Input: part model. Units: mm. Frame: model coordinates. Coordinates: 2 decimals unless noted, no trailing zeros. Order: outer loops, then holes, each group sorted by start corner. A loop starts at its lowest first (then second) coordinate and runs counter-clockwise, first axis right, second up.
from build123d import *

# Parameters (mm, degrees)
F0_W     = 25.4
F0_H     = 25.4
F2_R     = 19.05
F3_SIZE2 = 2.961044
F3_SIZE  = 6.34999


# Not quite as in the source:
# - a fillet or chamfer is up to 0.001 mm smaller than in the source, because OpenCascade refuses the exact size


with BuildPart() as f1:
    # F0 (on Front) → F1 (revolve)
    with BuildSketch(Plane.XZ):
        with Locations((12.7, 12.7)):
            Rectangle(F0_W, F0_H)
    revolve(axis=Axis((0, 0, 12.7), (0, 0, 1)))

    # F2
    f2_edges = [f1.edges().sort_by_distance(p)[0] for p in [
        (-25.4, 0, 25.4),
    ]]
    fillet(f2_edges, radius=F2_R)

    # F3 (size 6.35 and 2.9610536293 in the source; OpenCascade refuses exactly that, so slightly less here)
    f3_edges = [f1.edges().sort_by_distance(p)[0] for p in [
        (-25.4, 0, 0),
    ]]
    chamfer(f3_edges, length=F3_SIZE, length2=F3_SIZE2)


solid = f1.part
Item 1: Pin query (flat end, axial travel): pin 1 Ø2 at (x, z) = (-18.5, 17.5) entering from +Y; pin 2 Ø6 at (x, y) = (9, 8) entering from +Z; pin 3 Ø1 at (y, z) = (3.5, 6) entering from -X. Return the tip coordinate at first contact, or that it passes through.
Response values:
pin 1: stops at y = 13.42
pin 2: stops at z = 25.21
pin 3: stops at x = -25.2
Item 2: Cut plane A-A on z = 3.5. Return loops of the section in (x, y).
Response values:
outline: circle Ø48.14 at (0, 0)
Item 3: Ray query, probe 1 along Z at (x, y) = (15.5, -1); probe 2 along X at (y, z) = (-11.5, 17.5); probe 3 along Y at (x, z) = (-5, 20.25). Return the intervals inside material, ascending.
Response values:
probe 1: z = 0 to 23.04
probe 2: x = -18.52 to 18.52
probe 3: y = -18.72 to 18.72
